Check sheet for the modelled part. Datum: model origin and axes. Units: mm. A direction names the side the tool comes from. Give positions to 0.01 mm unless a question says otherwise; leave off trailing zeros. Order: outer loops, then holes, each group sorted by start corner. A loop starts at its lowest first (then second) coordinate and runs counter-clockwise, first axis right, second up. Notation, with made-up numbers: (79, 19.25) -> (114, 19.25) arc R27 ccw to (114, 52.25) -> close; hole circle Ø8 at (88, -21.75). An arc over 180 degrees is marked (long way). Answer in a Markdown table with one row per item. Add a question column.
(1) Cross-section at C-C (y = -101.6). Record the cut outline in (x, z).
(2) Go/stop test with flat-tipped pins: pin 1 (1.5 mm diameter, centred on y = -144.5, z = -27, fed in from +X); pin 2 (3 mm diameter, centred on y = -76.5, z = -29, fed in from +X); pin 3 (8 mm diameter, centred on y = -36, z = -13.5, fed in from +X). Record where each tip stops, or that it passes through.
(3) Set-up check for faces 1 (the face through (-52, -103, -1.27)), 2 (the face through (-26, -201.93, -29)), 3 (the face through (-47.617, -50.032, -0.626)): record each of +Z, -Z, +X, -X, +Y, -Y from which the full face is reachable in a straight line by a thin tool's end or side.
(4) Thickness scan on L1, parallel to Y at x = -37.5, z = -55; L2, parallel to Y at x = -61, z = -18; L3, parallel to Z at x = -47.5, y = -87.5. Record the ranges inside material, lowest first. Write a range as [from, to].
(5) Cross-section at D-D (z = -44.5). Record the cut outline in (x, y).
(6) Cross-section at B-B (x = -7). Record the cut outline in (y, z) (3 decimals).
(7) Release check for a two-part mould opening along Y. For faces 4 (the face through (-61.116, -199.919, -28.175)), 5 (the face through (-60.325, -4.274, -28.819)), 6 (the face through (0, -1, -20)), 7 (the face through (-13, -102, -10.16)) record: released by +Y, released by -Y, zero draft, split by the parting line, or undercut.
(8) Cross-section at A-A (z = -5.5). Record the cut outline in (x, y), then the cut area to 3 significant figures.
```python
from build123d import *

# Parameters (mm, degrees)
SKETCH1_W           = 114.3
SKETCH1_H           = 203.2
BOSS_EXTRUDE1_DEPTH = 88.9
CUT_EXTRUDE1_DEPTH  = 115.3
FILLET1_R           = 25.24
FILLET2_R           = 15.08
CUT_EXTRUDE2_DEPTH  = 115.3
LPATTERN1_COUNT     = 2
LPATTERN1_PITCH     = 101.6
SHELL5_T            = -1.27
SKETCH9_R           = 3
BOSS_EXTRUDE2_DEPTH = 8.89
SKETCH10_W          = 88.123203502
SKETCH10_H          = 57.15
CUT_EXTRUDE3_DEPTH  = 204.2


with BuildPart() as part:
    # Sketch1 → Boss-Extrude1 (new body)
    with BuildSketch(Plane(origin=(0, 0, 0), x_dir=(0, 0, -1), z_dir=(1, 0, 0))):
        with Locations((57.15, -101.6)):
            Rectangle(SKETCH1_W, SKETCH1_H)
    extrude(amount=-BOSS_EXTRUDE1_DEPTH)

    # Sketch4 → Cut-Extrude1 (cut, through all)
    with BuildSketch(Plane(origin=(0, 0, -114.3), x_dir=(-1, 0, 0), z_dir=(0, 0, -1))):
        Polygon((88.9, 0), (63.5, 0), (88.9, -101.6), align=None)
        Polygon((88.9, -203.2), (88.9, -101.6), (63.5, -203.2), align=None)
    extrude(amount=-CUT_EXTRUDE1_DEPTH, mode=Mode.SUBTRACT)

    # Fillet1
    fillet1_edges = [part.edges().sort_by_distance(p)[0] for p in [
        (-88.9, -101.6, -57.15),
    ]]
    fillet(fillet1_edges, radius=FILLET1_R)

    # Fillet2
    fillet2_edges = [part.edges().sort_by_distance(p)[0] for p in [
        (-63.5, 0, -57.15),
        (-63.5, -203.2, -57.15),
    ]]
    fillet(fillet2_edges, radius=FILLET2_R)

    # Sketch5 → Cut-Extrude2 (cut, through all)
    with BuildSketch(Plane.XY):
        with BuildLine():
            Line((-12.7, -187.325), (0, -187.325))
            Line((0, -187.325), (0, -117.475))
            Line((0, -117.475), (-12.7, -117.475))
            ThreePointArc((-12.7, -117.475), (-47.625, -152.4), (-12.7, -187.325))
        make_face()
    cut_extrude2 = extrude(amount=-CUT_EXTRUDE2_DEPTH, mode=Mode.SUBTRACT)

    # LPattern1: Cut-Extrude2 ×2
    with Locations(*[(0, i * LPATTERN1_PITCH, 0) for i in range(1, LPATTERN1_COUNT)]):
        add(cut_extrude2, mode=Mode.SUBTRACT)

    # Shell5
    shell5_openings = [part.faces().sort_by_distance(p)[0] for p in [
        (0, -195.2625, -57.15),
        (0, -101.6, -57.15),
        (-30.1625, -152.4, -57.15),
        (-6.35, -117.475, -57.15),
        (-6.35, -187.325, -57.15),
        (0, -7.9375, -57.15),
        (-30.1625, -50.8, -57.15),
        (-6.35, -15.875, -57.15),
        (-6.35, -85.725, -57.15),
    ]]
    offset(amount=SHELL5_T, openings=shell5_openings, kind=Kind.INTERSECTION)

    # Sketch9 → Boss-Extrude2 (add)
    with BuildSketch(Plane.XY.offset(-113.03)):
        with Locations((-12.7, -101.6)):
            Circle(SKETCH9_R)
    boss_extrude2 = extrude(amount=BOSS_EXTRUDE2_DEPTH)

    # Mirror1: Boss-Extrude2 across plane
    add(boss_extrude2.mirror(Plane.XY.offset(-57.15)))

    # Sketch10 → Cut-Extrude3 (cut, through all)
    with BuildSketch(Plane(origin=(0, 0, 0), x_dir=(1, 0, 0), z_dir=(0, 1, 0))):
        with Locations((-44.061601751, 85.725)):
            Rectangle(SKETCH10_W, SKETCH10_H)
    extrude(amount=-CUT_EXTRUDE3_DEPTH, mode=Mode.SUBTRACT)


solid = part.part
```
Answer below:
| question | item | result |
|---|---|---|
| 1 | outline | (-88.12, -57.15) -> (-86.85, -57.15) -> (-86.85, -1.27) -> (-15.7, -1.27) -> (-15.7, -10.16) -> (-9.7, -10.16) -> (-9.7, -1.27) -> (0, -1.27) -> (0, 0) -> (-88.12, 0) -> close |
| 2 | pin 1 | stops at x = -76.68 |
| 2 | pin 2 | stops at x = -80.94 |
| 2 | pin 3 | stops at x = -70.19 |
| 3 | face 1 | -Z |
| 3 | face 2 | -Z, +X |
| 3 | face 3 | +Z, -Z, +X |
| 4 | L1 | y = [-203.2, -201.93], [-1.27, 0] |
| 4 | L2 | y = [-200.01, -198.35], [-4.85, -3.19] |
| 4 | L3 | z = [-1.27, 0] |
| 5 | outline | (-87.37, -107.72) -> (-66.36, -191.78) arc R15.08 ccw to (-51.73, -203.2) -> (0, -203.2) -> (0, -201.93) -> (-51.73, -201.93) arc R13.81 cw to (-65.12, -191.47) -> (-86.14, -107.41) arc R23.97 cw to (-86.14, -95.79) -> (-65.12, -11.73) arc R13.81 cw to (-51.73, -1.27) -> (0, -1.27) -> (0, 0) -> (-51.73, 0) arc R15.08 ccw to (-66.36, -11.42) -> (-87.37, -95.48) arc R25.24 ccw to start |
| 6 | outline | (-203.2, -57.15) -> (-201.93, -57.15) -> (-201.93, -1.27) -> (-187.325, -1.27) -> (-187.325, 0) -> (-203.2, 0) -> close; (-117.475, -1.27) -> (-85.725, -1.27) -> (-85.725, 0) -> (-117.475, 0) -> close; (-15.875, -1.27) -> (-1.27, -1.27) -> (-1.27, -57.15) -> (0, -57.15) -> (0, 0) -> (-15.875, 0) -> close |
| 7 | face 4 | released by -Y |
| 7 | face 5 | undercut |
| 7 | face 6 | zero draft |
| 7 | face 7 | undercut |
| 8 | outline | (-87.37, -107.72) -> (-66.36, -191.78) arc R15.08 ccw to (-51.73, -203.2) -> (0, -203.2) -> (0, -201.93) -> (-51.73, -201.93) arc R13.81 cw to (-65.12, -191.47) -> (-86.14, -107.41) arc R23.97 cw to (-86.14, -95.79) -> (-65.12, -11.73) arc R13.81 cw to (-51.73, -1.27) -> (0, -1.27) -> (0, 0) -> (-51.73, 0) arc R15.08 ccw to (-66.36, -11.42) -> (-87.37, -95.48) arc R25.24 ccw to start; circle Ø6 at (-12.7, -101.6) |
| 8 | area | 444 mm² |
